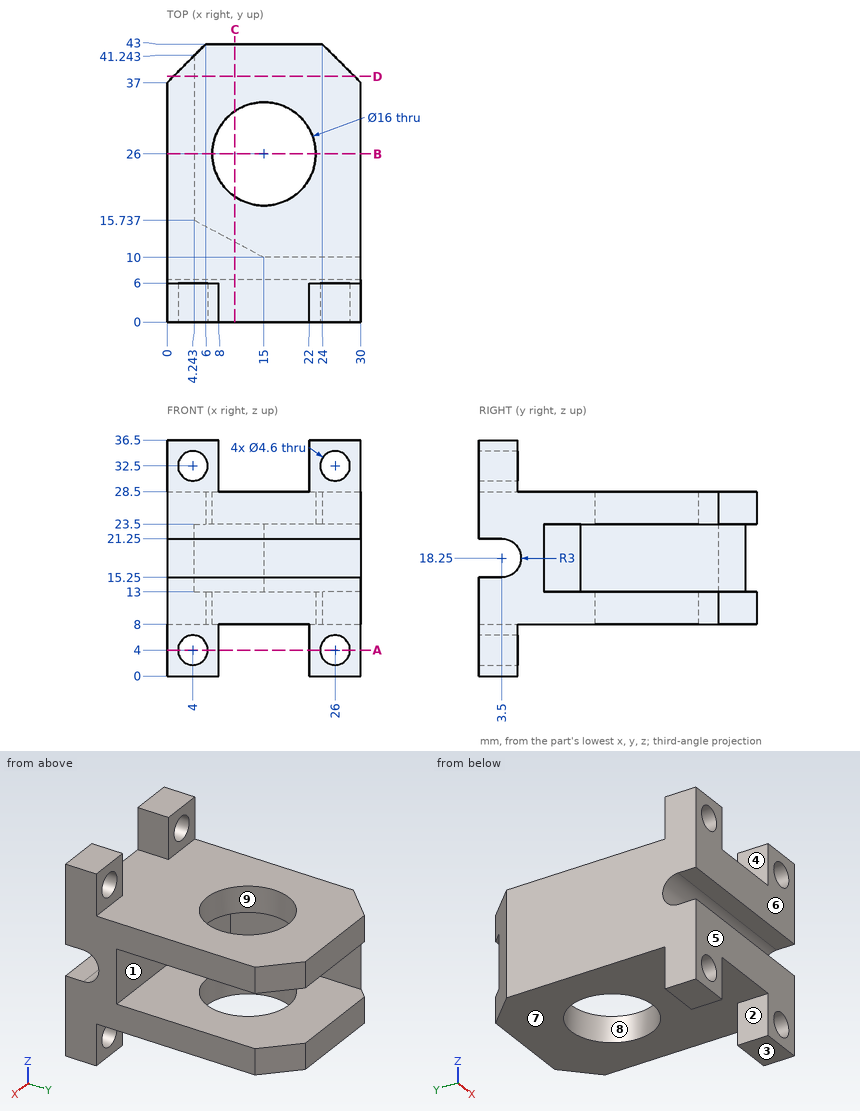
Geometry check sheet. Reference: drawing and pictorial views, mm from the part's lowest x, y, z. A direction names the side the tool comes from. Coordinates: 2 decimals unless noted, no trailing zeros. Write each loop counter-clockwise with the first axis right and the second up, starting at its lowest first coordinate (ties: lowest second). Pieces come first, ordered by that corner, then holes. Notation, with made-up numbers: M 27.5,8 L 56.5,8 A25 cw 56.5,25 Z; hole C -10,-9.75 d6. An arc over 180 degrees is marked long. Write item = value, one per line. Start each with the question number.
1. Sectioned sample at C-C (x = 10.5). State how many separate pieces and enclosed holes the cut face has, then the cut area to 3 significant figures.
2. Mould release check, pull along Y, two halves, no side actions. Record for the marked faces 6, 7, 8 and 9: pulls with the +Y half, pulls with the -Y half, needs draft (parallel to the pull), parting line crosses it, or undercut.
3. Sectioned sample at B-B (y = 26). Record the cut outline in (x, z).
4. Thickness scan on probe 1 along X at (y, z) = (4.75, 32.5); probe 2 along X at (y, z) = (26, 12); probe 3 along Z at (x, y) = (6, 39.5). Record the ranges inside material, lowest first.
5. Sectioned sample at D-D (y = 38). Record the cut outline in (x, z), then the cut area to 3 significant figures.
6. Tool access check on the marked faces 1, 2, 3, 4 and 5. Record the directions out of +Z, -Z, +X, -X, +Y, -Y that give a thin tool (end or side, any length) a straight path to the whole face; none if there is none.
7. Sectioned sample at A-A (z = 4). Record the cut outline in (x, y).
8. Go/stop test with flat-tipped pins: pin 1 (4 mm diameter, centred on x = 3, z = 31.5, fed in from +Y); pin 2 (5 mm diameter, centred on x = 19, z = 16.5, fed in from +Y); pin 3 (1 mm diameter, centred on x = 16, y = 2, fed in from +Z). Record where each tip stops, or that it passes through.
The answers:
q1.separate_pieces = 3
q1.enclosed_holes = 0
q1.area = 393 mm²
q2.face_6 = pulls with the -Y half
q2.face_7 = needs draft
q2.face_8 = undercut
q2.face_9 = undercut
q3.outline = M 0,8 L 7,8 L 7,13 L 4.24,13 L 4.24,23.5 L 7,23.5 L 7,28.5 L 0,28.5 Z; M 23,8 L 30,8 L 30,13 L 23,13 Z; M 23,23.5 L 30,23.5 L 30,28.5 L 23,28.5 Z
q4.probe_1 = 0 to 1.7, 6.3 to 8, 22 to 23.7, 28.3 to 30
q4.probe_2 = 0 to 7, 23 to 30
q4.probe_3 = 8 to 13, 23.5 to 28.5
q5.outline = M 1,8 L 29,8 L 29,13 L 4.24,13 L 4.24,23.5 L 29,23.5 L 29,28.5 L 1,28.5 Z
q5.area = 314 mm²
q6.face_1 = +X, +Y
q6.face_2 = -Z, +Y, -Y
q6.face_3 = -Z, +X, -X, +Y, -Y
q6.face_4 = +Z, +Y, -Y
q6.face_5 = +Z, -Z, +X, -X, -Y
q7.outline = M 0,0 L 1.7,0 L 1.7,6 L 0,6 Z; M 6.3,0 L 8,0 L 8,6 L 6.3,6 Z; M 22,0 L 23.7,0 L 23.7,6 L 22,6 Z; M 28.3,0 L 30,0 L 30,6 L 28.3,6 Z
q8.pin_1 = 6
q8.pin_2 = 10
q8.pin_3 = 28.5
